Can you work these out from the model? Positions are in its coordinate system, mm. A direction names the side the tool comes from. Give positions to 0.01 mm unless a question says otherwise; leave off trailing zeros. Loops run counter-clockwise (first coordinate to the right, second up) from the corner with the lowest first, then second, coordinate; pieces in that order, holes last. Notation, with made-up numbers: (-3, 56.5) -> (46, 56.5) arc R27 ccw to (46, 91.5) -> close; hole circle Ø10 at (46.5, 12). An arc over 180 degrees is marked (long way). One line per question, with ' | ' between items.
Autodesk Inventor part; units mm, degrees
ref_plane "YZ Plane" through (0, 0, 0) normal (1, 0, 0) x (0, 1, 0)
ref_plane "XZ Plane" through (0, 0, 0) normal (0, 1, 0) x (-1, 0, 0)
ref_plane "XY Plane" through (0, 0, 0) normal (0, 0, 1) x (1, 0, 0)
sketch "Sketch1" plane through (0, 0, 0) normal (0, 1, 0) x (-1, 0, 0)
  line L0 (0, 0) -> (26, 0)
  line L1 (26, 0) -> (26, -48)
  line L2 (26, -48) -> (0, -48)
  line L3 (0, -48) -> (0, 0)
  dimension "d0" = 26
  dimension "d1" = 48
extrude "Extrusion1" add sketch "Sketch1" along normal blind 32
sketch "Sketch2" plane through (0, 32, 0) normal (0, 1, 0) x (1, 0, 0)
  circle A0 centre (-13, 11.5) radius 3.5
  line L0 (0, 0) -> (-26, 0)
  line L1 (0, 0) -> (0, 48)
  dimension "d4" = 7
  dimension "d5" = 11.5
  dimension "d6" = 26
  dimension "d7" = 13
extrude "Extrusion2" cut sketch "Sketch2" against normal blind 10
sketch "Sketch3" plane through (0, 0, 0) normal (1, 0, 0) x (0, 0, -1)
  line L0 (0, 32) -> (48, 32)
  line L1 (14.75, 32) -> (45.25, 32)
  line L2 (45.25, 32) -> (45.25, 27)
  line L3 (45.25, 27) -> (14.75, 27)
  line L4 (14.75, 27) -> (14.75, 32)
  line L5 (48, 0) -> (0, 0)
  line L6 (45.25, 0) -> (14.75, 0)
  line L7 (14.75, 0) -> (14.75, 5)
  line L8 (14.75, 5) -> (45.25, 5)
  line L9 (45.25, 5) -> (45.25, 0)
  line L10 (0, 0) -> (0, 32)
  line L11 (48, 0) -> (48, 32)
  dimension "d10" = 5
  dimension "d11" = 5
  dimension "d12" = 30.5
  dimension "d13" = 30.5
  dimension "d52" = 14.75
extrude "Extrusion3" add sketch "Sketch3" along normal blind 2 contours L0 L2 L3 L4 | L7 L8 L9 L5
sketch "Sketch4" plane through (-26, 0, -48) normal (-1, 0, 0) x (0, 0, 1)
  line L0 (2.75, 27) -> (2.75, 32)
  line L1 (2.75, 32) -> (33.25, 32)
  line L2 (33.25, 32) -> (33.25, 27)
  line L3 (33.25, 27) -> (2.75, 27)
  line L4 (2.75, 27) -> (2.75, 32)
  line L5 (33.25, 0) -> (2.75, 0)
  line L6 (2.75, 0) -> (2.75, 5)
  line L7 (2.75, 5) -> (33.25, 5)
  line L8 (33.25, 5) -> (33.25, 0)
  point P0 (48, 0)
extrude "Extrusion4" add sketch "Sketch4" along normal blind 2
sketch "Sketch5" plane through (0, 32, 0) normal (0, 1, 0) x (1, 0, 0)
  circle A0 centre (0.5, 42) radius 1
  line L0 (0, 45.25) -> (2, 45.25)
  line L1 (2, 45.25) -> (2, 14.75)
  circle A1 centre (-13, 11.5) radius 3.5
  line L2 (-26, 0) -> (0, 0)
  line L3 (0, 0) -> (0, 14.75)
  line L4 (0, 14.75) -> (2, 14.75)
  line L5 (2, 45.25) -> (2, 14.75)
  line L6 (0, 45.25) -> (2, 45.25)
  line L7 (0, 48) -> (-26, 48)
  line L8 (-26, 48) -> (-26, 45.25)
  line L9 (-26, 45.25) -> (-28, 45.25)
  line L10 (-28, 14.75) -> (-28, 45.25)
  line L11 (-26, 14.75) -> (-28, 14.75)
  circle A2 centre (0.5, 34) radius 1
  circle A3 centre (0.5, 26) radius 1
  circle A4 centre (0.5, 18) radius 1
  circle A5 centre (-26.5, 42) radius 1
  circle A6 centre (-26.5, 34) radius 1
  circle A7 centre (-26.5, 26) radius 1
  circle A8 centre (-26.5, 18) radius 1
  line L12 (0, 45.25) -> (0, 48)
  line L13 (-26, 14.75) -> (-26, 0)
  point P0 (0, 48.5)
  dimension "d20" = 2
  dimension "d21" = 3.25
  dimension "d24" = 8
  dimension "d29" = 3.25
  dimension "d30" = 1.5
  dimension "d32" = 2
  dimension "d33" = 1.5
  dimension "d36" = 8
  dimension "d41" = 3.25
  dimension "d42" = 3.25
extrude "Extrusion5" cut sketch "Sketch5" against normal through all contours A0 | A2 | A3 | A4 | A5 | A6 | A7 | A8
equation "\"d7\" = 0.5 * d6"
equation "\"d10\" = d11"
equation "\"d21\" = d29"
equation "\"d41\" = d42"
properties part number "ax12" material "ABS Plastic"
Q1. If we section it at C-C (z = -37): Write out the boundary of the cut face in (x, y).
Entries:
outline: (-28, 0) -> (2, 0) -> (2, 5) -> (0, 5) -> (0, 27) -> (2, 27) -> (2, 32) -> (-28, 32) -> (-28, 27) -> (-26, 27) -> (-26, 5) -> (-28, 5) -> close
Q2. For pin 1 Ø1.6 at (x, y) = (-27, 3) entering from -Z; pin 2 Ø6 at (y, z) = (8.5, -23.5) entering from -X; pin 3 Ø3.5 at (x, z) = (-13.5, -13) entering from +Y; pin 4 Ø1.6 at (x, z) = (0.5, -18) entering from -Y, each with a flat end and sliding along its axis, tell me the tip position at first contact or that it passes through.
Entries:
pin 1: z = -45.25 | pin 2: x = -26 | pin 3: y = 22 | pin 4: through
Q3. If we section it at A-A (z = -18): Write out the boundary of the cut face in (x, y), plus the area to 3 significant figures.
Entries:
outline: (-28, 0) -> (-27.5, 0) -> (-27.5, 5) -> (-28, 5) -> close; (-28, 27) -> (-27.5, 27) -> (-27.5, 32) -> (-28, 32) -> close; (-25.5, 0) -> (-0.5, 0) -> (-0.5, 32) -> (-25.5, 32) -> close; (1.5, 0) -> (2, 0) -> (2, 5) -> (1.5, 5) -> close; (1.5, 27) -> (2, 27) -> (2, 32) -> (1.5, 32) -> close | area: 810 mm²
Q4. On a 3-axis mill with a long thin cutter (end or side, diameter ignored), from which of +Z, -Z, +X, -X, +Y, -Y can I reach the whole of each face in a straight line? I mean faces 1 (the face through (-26, 16, -22)), 2 (the face through (-27, 30, -14.75)), 3 (the face through (0, 16, -30)), 4 (the face through (-27, 29, -45.25)). Say none if no direction works.
Entries:
face 1: +Z, -Z, -X | face 2: +Z, -X, +Y, -Y | face 3: +Z, -Z, +X | face 4: -Z, -X, +Y, -Y
Q5. If we mould it in two halves opening along Z, with no side actions, what happens to faces 5 (the face through (-13, 32, -24)), 6 (the face through (-13, 22, -12)), 7 (the face through (1, 30, -45.25))? For each: pulls with the +Z half, pulls with the -Z half, needs draft (parallel to the pull), parting line crosses it, or undercut.
Entries:
face 5: needs draft | face 6: undercut | face 7: pulls with the -Z half
Q6. If we section it at B-B (y = 29): State how many separate pieces and enclosed holes the cut face has, plus the area to 3 significant figures.
Entries:
separate pieces: 1 | enclosed holes: 9 | area: 1,310 mm²
Q7. If we section it at D-D (y = 8.5): Write out the boundary of the cut face in (x, z), plus the area to 3 significant figures.
Entries:
outline: (-26, -48) -> (0, -48) -> (0, -42.87) arc R1 cw to (0, -41.13) -> (0, -34.87) arc R1 cw to (0, -33.13) -> (0, -26.87) arc R1 cw to (0, -25.13) -> (0, -18.87) arc R1 cw to (0, -17.13) -> (0, 0) -> (-26, 0) -> (-26, -17.13) arc R1 cw to (-26, -18.87) -> (-26, -25.13) arc R1 cw to (-26, -26.87) -> (-26, -33.13) arc R1 cw to (-26, -34.87) -> (-26, -41.13) arc R1 cw to (-26, -42.87) -> close | area: 1,240 mm²
Q8. If I drill on probe 1 along Z at (x, y) = (-13, 29); probe 2 along X at (y, z) = (30.25, -11.5); probe 3 along X at (y, z) = (11, -18), over which ranges is the centre line in solid material (lowest first)? Write a range as from..to.
Entries:
probe 1: -48..-15, -8..0 | probe 2: -26..-16.5, -9.5..0 | probe 3: -25.5..-0.5
